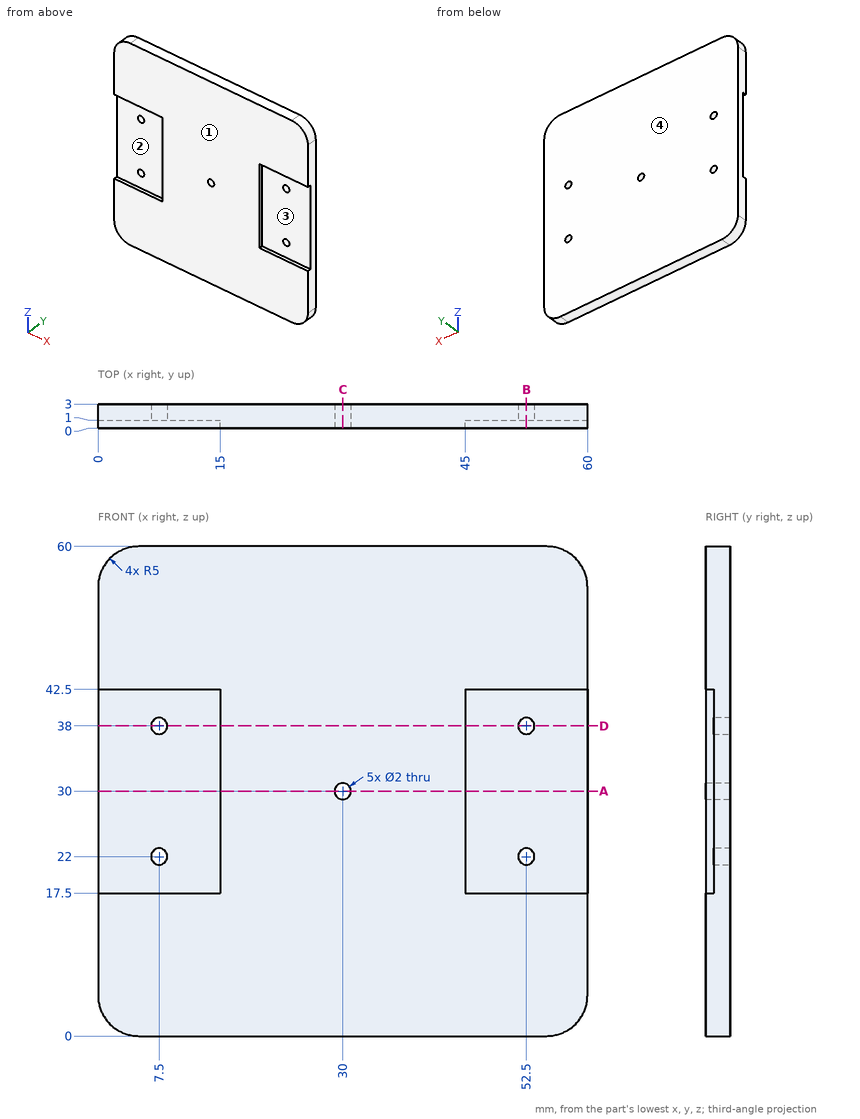
Study the drawing (mm; zero at the part's minimum x, y, z) and answer. A direction names the side the tool comes from. Round coordinates to 2 decimals unless told otherwise and drop trailing zeros. Write each loop counter-clockwise with the first axis right and the second up, starting at its lowest first coordinate (ties: lowest second). Pieces come first, ordered by that corner, then holes. Notation, with made-up numbers: (72, 48) - (124, 48) arc R29 cw to (124, 74) - close; hole circle Ø9 at (22, 5.25). An arc over 180 degrees is marked (long way). Use a Markdown table: item, result. Add a question column.
1. The part is cut by section A-A (z = 30). Write down the section's boundary in (x, y).
2. The part is cut by section D-D (z = 38). Write down the section's boundary in (x, y), and give its area (3 significant figures).
3. The part is cut by section B-B (x = 52.5). Write down the section's boundary in (y, z), and give its area (3 significant figures).
4. For a pull along Z with two mould halves and no side action, classify the marked faces 1 and 2 as +Z half, -Z half, draft (parallel to the pull), parting line (faces both ways), or undercut.
5. A tool of negligible diameter and unlimited length cuts with its end or side. For the marked faces 3 and 4, from which of +Z, -Z, +X, -X, +Y, -Y can it reach the whole face along a straight path? Write none if from no direction.
6. The part is cut by section C-C (x = 30). Write down the section's boundary in (y, z), and give its area (3 significant figures).
7. Flat-ended cylindrical pins translate along their axes: P1, Ø4.5, axis at x = 5, z = 30, coming from the -Y side; P2, Ø1.8, axis at x = 7.5, z = 22, coming from the +Y side; P3, Ø0.5, axis at y = 0.5, z = 35.5, coming from the +X side. Find the tip coordinate at first contact, or state that the pin passes through.
8. Consider line 1 (X direction, y = 1.9, z = 22); line 2 (Z direction, x = 13, y = 0.5); line 3 (Y direction, x = 51, z = 23.5). Determine where each line is inside the solid, lowest interval first.
Reported:
| question | item | result |
|---|---|---|
| 1 | outline | (0, 1) - (15, 1) - (15, 0) - (29, 0) - (29, 3) - (0, 3) - close; (31, 0) - (45, 0) - (45, 1) - (60, 1) - (60, 3) - (31, 3) - close |
| 2 | outline | (0, 1) - (6.5, 1) - (6.5, 3) - (0, 3) - close; (8.5, 1) - (15, 1) - (15, 0) - (45, 0) - (45, 1) - (51.5, 1) - (51.5, 3) - (8.5, 3) - close; (53.5, 1) - (60, 1) - (60, 3) - (53.5, 3) - close |
| 2 | area | 142 mm^2 |
| 3 | outline | (0, 0) - (3, 0) - (3, 21) - (1, 21) - (1, 17.5) - (0, 17.5) - close; (0, 42.5) - (1, 42.5) - (1, 39) - (3, 39) - (3, 60) - (0, 60) - close; (1, 23) - (3, 23) - (3, 37) - (1, 37) - close |
| 3 | area | 147 mm^2 |
| 4 | face 1 | draft |
| 4 | face 2 | undercut |
| 5 | face 3 | +X, -Y |
| 5 | face 4 | +Z, -Z, +X, -X, +Y |
| 6 | outline | (0, 0) - (3, 0) - (3, 29) - (0, 29) - close; (0, 31) - (3, 31) - (3, 60) - (0, 60) - close |
| 6 | area | 174 mm^2 |
| 7 | P1 | y = 1 |
| 7 | P2 | through |
| 7 | P3 | x = 45 |
| 8 | line 1 | 0 to 6.5, 8.5 to 51.5, 53.5 to 60 |
| 8 | line 2 | 0 to 17.5, 42.5 to 60 |
| 8 | line 3 | 1 to 3 |
